Source: CAD feature listing. Evaluate the final solid. Frame: model axes, mm. Give positions to 0.01 mm unless a question says otherwise; leave off trailing zeros. Order: outer loops, then holes, each group sorted by start corner. A loop starts at its lowest first (then second) coordinate and runs counter-clockwise, first axis right, second up. Notation, with made-up numbers: M 71.5,-29.75 L 127.5,-29.75 A15 cw 127.5,-8.75 Z; hole C 33.25,9.5 d4. An arc over 180 degrees is marked long. Return JSON: item names as keys, results as strings.
from build123d import *

# Parameters (mm, degrees)
F0_W     = 952.5
F0_H     = 127
F1_DEPTH = 19.05
F3_DEPTH = 952.501
F5_DEPTH = 127.0010001


with BuildPart() as f1:
    # F0 (on Front) → F1 (new body)
    with BuildSketch(Plane.XZ):
        Rectangle(F0_W, F0_H)
    extrude(amount=F1_DEPTH)

    # F2 (on face) → F3 (cut, through all)
    with BuildSketch(Plane.YZ.offset(476.25)):
        with BuildLine():
            add(Edge.make_bspline(
                [(0, 63.5), (-13.8609133718, 63.5), (-9.1129885479, 55.0204556119), (-15.256598862, 52.3182653746)],
                knots=[0, 0, 0, 0, 19.4568359991, 19.4568359991, 19.4568359991, 19.4568359991], degree=3))
            Line((0, 63.5), (-19.05, 63.5))
            Line((-19.05, 63.5), (-19.05, 51.528967917))
            add(Edge.make_bspline(
                [(-15.256598862, 52.3182653746), (-16.2172018341, 51.8957561593), (-17.4440793365, 51.6144907855), (-19.05, 51.528967917)],
                knots=[19.4568359991, 19.4568359991, 19.4568359991, 19.4568359991, 22.4990690726, 22.4990690726, 22.4990690726, 22.4990690726], degree=3))
        make_face()
        with BuildLine():
            ThreePointArc((-19.05, 46.505666794), (-18.0177487141, 49.976120455), (-15.256598862, 52.3182653746))
            add(Edge.make_bspline(
                [(-15.256598862, 52.3182653746), (-16.2172018341, 51.8957561593), (-17.4440793365, 51.6144907855), (-19.05, 51.528967917)],
                knots=[19.4568359991, 19.4568359991, 19.4568359991, 19.4568359991, 22.4990690726, 22.4990690726, 22.4990690726, 22.4990690726], degree=3))
            Line((-19.05, 51.528967917), (-19.05, 46.505666794))
        make_face()
    extrude(amount=-F3_DEPTH, mode=Mode.SUBTRACT)

    # F4 (on face) → F5 (cut, through all)
    with BuildSketch(Plane(origin=(0, 0, -63.5), x_dir=(1, 0, 0), z_dir=(0, 0, -1))):
        Polygon((-457.2, 0), (-476.25, 19.05), (-476.25, 0), align=None)
        Polygon((476.25, 19.05), (457.2, 0), (476.25, 0), align=None)
    extrude(amount=-F5_DEPTH, mode=Mode.SUBTRACT)


solid = f1.part
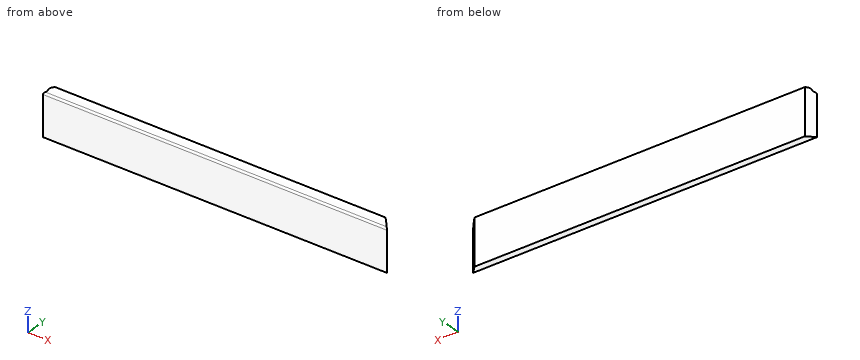
1. Ray query, probe 1 along Z at (x, y) = (-387, -15); probe 2 along X at (y, z) = (-15.25, -57); probe 3 along Z at (x, y) = (-291, -1.25). Return the intervals inside material, ascending.
Evaluation:
{"probe 1": "z = -63.5 to 52.44", "probe 2": "x = -472.45 to 472.45", "probe 3": "z = -63.5 to 63.48"}
2. Section query A-A (z = 36). Return loops of the section in (x, y), then the cut area to 3 significant figures.
Evaluation:
{"outline": "M -476.25,-19.05 L 476.25,-19.05 L 457.2,0 L -457.2,0 Z", "area": "17,800 mm^2"}
3. First-contact query: pin 1 (5 mm diameter, centred on y = -12.5, z = 37, fed in from -X); pin 2 (1 mm diameter, centred on y = -4.5, z = -23.5, fed in from -X); pin 3 (5 mm diameter, centred on y = -14, z = 15, fed in from +X); pin 4 (1 mm diameter, centred on x = 285.5, z = 0, fed in from +Y). Flat tips, straight axial feed; report the tip coordinate or a pass-through.
Evaluation:
{"pin 1": "stops at x = -472.2", "pin 2": "stops at x = -462.2", "pin 3": "stops at x = 473.7", "pin 4": "stops at y = 0"}
